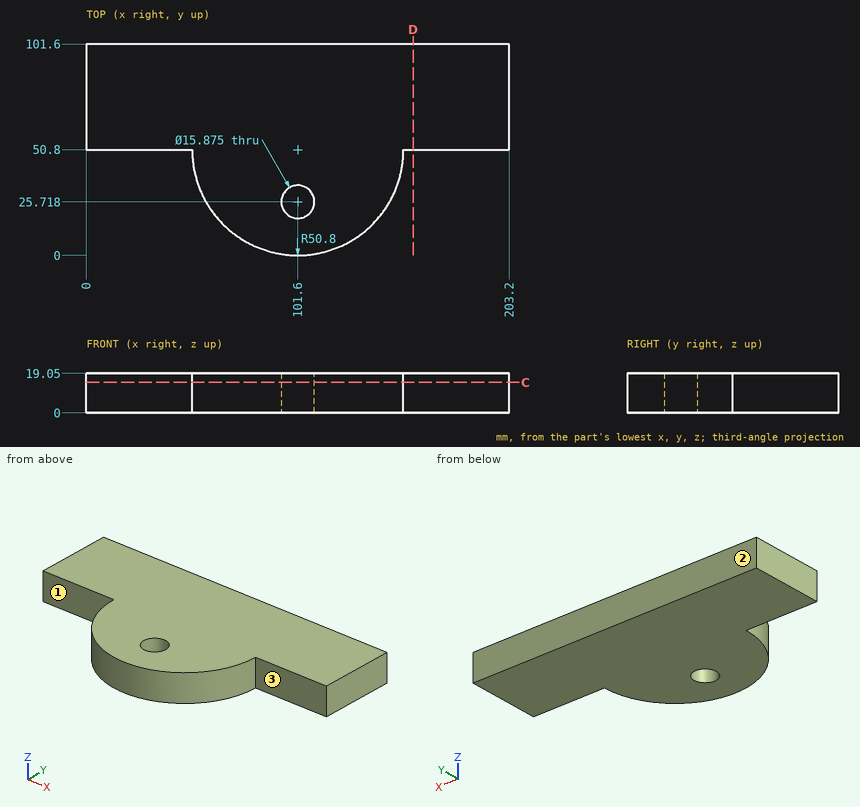
Could you check a few things on this drawing? It's one solid part, dimensions in mm from its lowest x, y, z. A direction names the side the tool comes from. Coordinates: 2 decimals unless noted, no trailing zeros. Loops run counter-clockwise (first coordinate to the right, second up) from the corner with the lowest first, then second, coordinate; pieces in that order, holes last.
1. For the marked faces 1, 2 and 3, which set-ups out of +Z, -Z, +X, -X, +Y, -Y let a thin tool reach every point of the face, with its end or its side?
2. Imagine slicing it at C-C (z = 14.75). Please give me the cut outline in (x, y) (1 decimal).
3. I need wall thicknesses on L1, parallel to Y at x = 101.6, z = 4.5 (1 decimal); L2, parallel to Y at x = 161.5, z = 16.25; L3, parallel to X at y = 22, z = 4.5 (1 decimal). Which ranges of each line are inside material? Lowest first, please.
4. For P1, Ø2, axis at y = 37.5, z = 2.5, coming from the -X side; P2, Ø5.5, axis at x = 13.5, z = 5.5, coming from the -Y side; P3, Ø8, axis at y = 30.5, z = 13, coming from the +X side; P4, Ø9.5, axis at x = 101.6, y = 25.72, coming from the -Z side, each with a flat end and sliding along its axis, tell me the tip position at first contact or that it passes through.
5. Imagine slicing it at D-D (x = 157). Please give me the cut outline in (y, z), and give its area (3 significant figures).
Computed values:
1. face 1: +Z, -Z, -X, -Y
1. face 2: +Z, -Z, +X, -X, +Y
1. face 3: +Z, -Z, +X, -Y
2. outline: (0, 50.8) - (50.8, 50.8) arc R50.8 ccw to (152.4, 50.8) - (203.2, 50.8) - (203.2, 101.6) - (0, 101.6) - close; hole circle Ø15.9 at (101.6, 25.7)
3. L1: y = 0 to 17.8, 33.7 to 101.6
3. L2: y = 50.8 to 101.6
3. L3: x = 59.8 to 94.6, 108.6 to 143.4
4. P1: stops at x = 52.31
4. P2: stops at y = 50.8
4. P3: stops at x = 149.71
4. P4: passes through
5. outline: (50.8, 0) - (101.6, 0) - (101.6, 19.05) - (50.8, 19.05) - close
5. area: 968 mm2
